CAD build for the part. Positions are in the model's coordinates, mm. A direction names the side the tool comes from. Round coordinates to 2 decimals unless told otherwise and drop trailing zeros. Order: outer loops, then holes, each group sorted by start corner. A loop starts at its lowest first (then second) coordinate and runs counter-clockwise, first axis right, second up.
```python
from build123d import *

# Parameters (mm, degrees)
SKETCH2_W           = 120
SKETCH2_H           = 400
THICKEN1_T1         = 10
SKETCH3_W           = 60
SKETCH3_H           = 20
BOSS_EXTRUDE1_DEPTH = 60
FILLET3_R           = 5
SKETCH5_R           = 1.5
CUT_EXTRUDE4_DEPTH  = 31
RIB1_REACH          = 226.778
SKETCH8_WALL_W      = 523.072195762
SKETCH8_WALL_H      = 6.5
FILLET4_R           = 2


with BuildPart() as body_1:
    # Sketch2 → Surface-Plane1: a flat surface bounded by the sketch
    with BuildSketch(Plane(origin=(0, 0, 0), x_dir=(1, 0, 0), z_dir=(0, 1, 0)), mode=Mode.PRIVATE) as surface_plane1_1_region:
        Rectangle(SKETCH2_W, SKETCH2_H)
    surface_plane1_1 = surface_plane1_1_region.sketch.faces()[0]
    add(Solid.thicken(surface_plane1_1, THICKEN1_T1))

    # Sketch3 → Boss-Extrude1 (add)
    with BuildSketch(Plane(origin=(0, 10, 0), x_dir=(1, 0, 0), z_dir=(0, 1, 0))):
        with Locations((0, -190)):
            Rectangle(SKETCH3_W, SKETCH3_H)
    extrude(amount=BOSS_EXTRUDE1_DEPTH)

    # Fillet3
    fillet3_edges = [body_1.edges().sort_by_distance(p)[0] for p in [
        (30, 10, 190),
        (-30, 10, 190),
    ]]
    fillet(fillet3_edges, radius=FILLET3_R)

    # Sketch5 → Cut-Extrude4 (cut)
    with BuildSketch(Plane.XY.offset(200)):
        with Locations((0, 50.5)):
            Circle(SKETCH5_R)
        with Locations((-8, 42.5)):
            Circle(SKETCH5_R)
        with Locations((0, 34.5)):
            Circle(SKETCH5_R)
        with Locations((8, 42.5)):
            Circle(SKETCH5_R)
    extrude(amount=-CUT_EXTRUDE4_DEPTH, mode=Mode.SUBTRACT)

    # Sketch8 wall → Rib1 (add, up to next)
    with BuildSketch(Plane(origin=(15, 40, 160.540675435), x_dir=(0, -0.838963009324, -0.544188449882), z_dir=(0, 0.544188449882, -0.838963009324)), mode=Mode.PRIVATE) as rib1_sk1:
        Rectangle(SKETCH8_WALL_W, SKETCH8_WALL_H)
    rib1_tool1 = extrude(rib1_sk1.sketch, amount=-RIB1_REACH, mode=Mode.PRIVATE) - body_1.part
    rib1 = rib1_tool1.solids().sort_by_distance((15, 40, 160.540675435))[0]
    add(rib1)

    # Mirror1: Rib1 across plane
    add(rib1.mirror(Plane(origin=(0, 0, 0), x_dir=(0, 0, 1), z_dir=(1, 0, 0))))

    # Fillet4
    fillet4_edges = [body_1.edges().sort_by_distance(p)[0] for p in [
        (-18.25, 10, 160.540675435),
        (-15, 10, 141.08135087),
        (-11.75, 10, 160.540675435),
        (0, 10, 180),
        (11.75, 10, 160.540675435),
        (15, 10, 141.08135087),
        (18.25, 10, 160.540675435),
        (26.625, 10, 180),
        (-18.25, 40, 180),
        (-11.75, 40, 180),
        (11.75, 40, 180),
        (18.25, 40, 180),
    ]]
    fillet(fillet4_edges, radius=FILLET4_R)


solid = body_1.part
```
1. Tool access for faces 1 (the face through (-11.75, 28, 166)), 2 (the face through (-60, 5, -3)), 3 (the face through (18.25, 28, 166)), 4 (the face through (-18.25, 28, 166)), 5 (the face through (-30, 42, 190)): list every direction of +Z, -Z, +X, -X, +Y, -Y with a clear straight run to the whole face (end or side of a thin tool).
2. Cut at D-D, the plane x = -51. Write the cut outline in (y, z).
3. Mould opens along X. For faces 6 (the face through (30, 42, 190)), 7 (the face through (0, 41, 180)), 8 (the face through (0, 70, 190)) say: released by +X, released by -X, zero draft, split by the parting line, or undercut.
4. Pin check, flat tips, straight feed: P1, Ø5.5, axis at x = 26, y = 52.5, coming from the -Z side; P2, Ø10.5, axis at y = 41.5, z = 162.5, coming from the -X side; P3, Ø22, axis at y = 35.5, z = 194, coming from the +X side. Stop position of each tip, or through.
5. Cut at B-B, the plane y = 60.5. Write the cut outline in (x, z).
6. Cut at C-C, the plane z = 136.5. Write the cut outline in (x, y), and give its area (3 significant figures).
7. Drill centre lines: line 1 (Y direction, x = 0, z = 193.25); line 2 (Y direction, x = 8, z = 196); line 3 (X direction, y = 42, z = 187). Where is each one in solid material? Low to high.
8. Cut at A-A, the plane x = 25.5. Write the cut outline in (y, z), and give its area (3 significant figures).
Outcome:
1. face 1: -Z, +Y
1. face 2: +Z, -Z, -X, +Y, -Y
1. face 3: -Z, +X, +Y
1. face 4: -Z, -X, +Y
1. face 5: +Z, -Z, -X, +Y
2. outline: (0, -200) - (10, -200) - (10, 200) - (0, 200) - close
3. face 6: released by +X
3. face 7: undercut
3. face 8: zero draft
4. P1: stops at z = 180
4. P2: stops at x = -18.25
4. P3: stops at x = 30
5. outline: (-30, 180) - (-20.25, 180) arc R2 cw to (-18.25, 178) - (-18.25, 173.84) - (-11.75, 173.84) - (-11.75, 178) arc R2 cw to (-9.75, 180) - (9.75, 180) arc R2 cw to (11.75, 178) - (11.75, 173.84) - (18.25, 173.84) - (18.25, 178) arc R2 cw to (20.25, 180) - (30, 180) - (30, 200) - (-30, 200) - close
6. outline: (-60, 0) - (60, 0) - (60, 10) - (-60, 10) - close
6. area: 1,200 mm2
7. line 1: y = 0 to 33, 36 to 49, 52 to 70
7. line 2: y = 0 to 41, 44 to 70
7. line 3: x = -30 to -9.41, -6.59 to 6.59, 9.41 to 30
8. outline: (0, -200) - (10, -200) - (10, 178) arc R2 cw to (12, 180) - (70, 180) - (70, 200) - (0, 200) - close
8. area: 5,200 mm2
